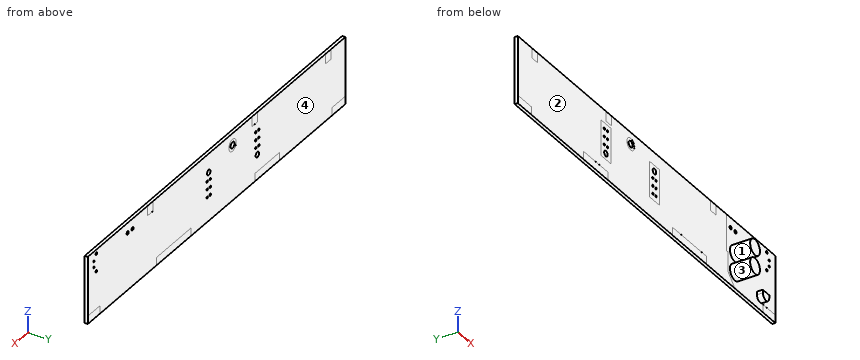
from build123d import *

# Parameters (mm, degrees)
ESQUISSE1_W                     = 210
ESQUISSE1_H                     = 1.6
BOARD_DEPTH                     = 34
SKETCH1_R                       = 0.55
SKETCH1_R_2                     = 1.4
REMOVEABLE_BATT_CON_HOLES_DEPTH = 118.625713289
SKETCH2_R                       = 0.51
SKETCH2_R_2                     = 0.635
DC_OUT_CONN_HOLES_DEPTH         = 118.625713289
SKETCH3_R                       = 0.85
CHARGER_CONN_HOLES_DEPTH        = 118.625713289
SKETCH4_R                       = 1.59
CUT_EXTRUDE1_DEPTH              = 118.625713289
SKETCH5_R                       = 3
SKETCH5_W                       = 10
SKETCH5_H                       = 4
SKETCH5_W_2                     = 28
SKETCH5_W_3                     = 20
SKETCH5_W_4                     = 11
SKETCH5_W_5                     = 4.5
SKETCH5_H_2                     = 5
CUT_EXTRUDE2_DEPTH              = 0.01
CUT_EXTRUDE3_START              = -1.59
SKETCH5_2_R                     = 3
SKETCH5_2_W                     = 10
SKETCH5_2_H                     = 4
SKETCH5_2_W_2                   = 28
SKETCH5_2_W_3                   = 20
SKETCH5_2_W_4                   = 11
SKETCH5_2_W_5                   = 4.5
SKETCH5_2_H_2                   = 5
CUT_EXTRUDE3_DEPTH              = 0.01
SKETCH6_W                       = 8
SKETCH6_H                       = 18
CUT_EXTRUDE4_DEPTH              = 0.001
SKETCH7_R                       = 4
BOSS_EXTRUDE1_DEPTH             = 10.2
BOSS_EXTRUDE2_DEPTH             = 3


with BuildPart() as part:
    # Esquisse1 → Board (new body)
    with BuildSketch(Plane.XY):
        with Locations((-7.593287663, -121.91)):
            Rectangle(ESQUISSE1_W, ESQUISSE1_H)
    extrude(amount=BOARD_DEPTH)

    # Sketch1 → Removeable Batt Con Holes (cut, through all)
    with BuildSketch(Plane(origin=(0, -122.71, 0), x_dir=(1, 0, 0), z_dir=(0, 1, 0))):
        with Locations(Location((-39.523287663, -16.5, 0), (0, 0, 180))):
            Circle(SKETCH1_R)
        with Locations(Location((-42.063287663, -16.5, 0), (0, 0, 180))):
            Circle(SKETCH1_R)
        with Locations(Location((-42.063287663, -20.5, 0), (0, 0, 180))):
            Circle(SKETCH1_R)
        with Locations(Location((-42.063287663, -24.5, 0), (0, 0, 180))):
            Circle(SKETCH1_R)
        with Locations((-40.793287663, -12.5)):
            Circle(SKETCH1_R_2)
        with Locations(Location((-39.523287663, -20.5, 0), (0, 0, 180))):
            Circle(SKETCH1_R)
        with Locations(Location((-39.523287663, -24.5, 0), (0, 0, 180))):
            Circle(SKETCH1_R)
        with Locations(Location((-2.463287663, -20.5, 0), (0, 0, 180))):
            Circle(SKETCH1_R)
        with Locations(Location((0.076712337, -20.5, 0), (0, 0, 180))):
            Circle(SKETCH1_R)
        with Locations(Location((-2.463287663, -16.5, 0), (0, 0, 180))):
            Circle(SKETCH1_R)
        with Locations(Location((0.076712337, -16.5, 0), (0, 0, 180))):
            Circle(SKETCH1_R)
        with Locations(Location((-2.463287663, -12.5, 0), (0, 0, 180))):
            Circle(SKETCH1_R)
        with Locations(Location((0.076712337, -12.5, 0), (0, 0, 180))):
            Circle(SKETCH1_R)
        with Locations((-1.193287663, -24.5)):
            Circle(SKETCH1_R_2)
    extrude(amount=REMOVEABLE_BATT_CON_HOLES_DEPTH, mode=Mode.SUBTRACT)

    # Sketch2 → DC Out Conn holes (cut, through all)
    with BuildSketch(Plane.XZ.offset(122.71)):
        with Locations((92.406712337, 29)):
            Circle(SKETCH2_R)
        with Locations((92.406712337, 26)):
            Circle(SKETCH2_R)
        with Locations((90.446712337, 32)):
            Circle(SKETCH2_R_2)
        with Locations((90.446712337, 23)):
            Circle(SKETCH2_R_2)
    extrude(amount=-DC_OUT_CONN_HOLES_DEPTH, mode=Mode.SUBTRACT)

    # Sketch3 → Charger conn holes (cut, through all)
    with BuildSketch(Plane.XZ.offset(122.71)):
        with Locations((64.906712337, 28.92)):
            Circle(SKETCH3_R)
        with Locations((60.946712337, 28.92)):
            Circle(SKETCH3_R)
    extrude(amount=-CHARGER_CONN_HOLES_DEPTH, mode=Mode.SUBTRACT)

    # Sketch4 → Cut-Extrude1 (cut, through all)
    with BuildSketch(Plane(origin=(0, -121.11, 0), x_dir=(1, 0, 0), z_dir=(0, 1, 0))):
        with Locations(Location((-20.593287663, -28, 0), (0, 0, 180))):
            Circle(SKETCH4_R)
    extrude(amount=-CUT_EXTRUDE1_DEPTH, mode=Mode.SUBTRACT)

    # Sketch5 → Cut-Extrude2 (cut)
    with BuildSketch(Plane(origin=(0, -121.11, 0), x_dir=(1, 0, 0), z_dir=(0, 1, 0))):
        with Locations(Location((-20.593287663, -28, 0), (0, 0, 180))):
            Circle(SKETCH5_R)
        with Locations((92.406712337, -2)):
            Rectangle(SKETCH5_W, SKETCH5_H)
        with Locations((27.406712337, -2)):
            Rectangle(SKETCH5_W_2, SKETCH5_H)
        with Locations((-49.093287663, -2)):
            Rectangle(SKETCH5_W_3, SKETCH5_H)
        with Locations((-107.093287663, -2)):
            Rectangle(SKETCH5_W_4, SKETCH5_H)
        with Locations((-98.743287663, -31.5)):
            Rectangle(SKETCH5_W_5, SKETCH5_H_2)
        with Locations((-38.543287663, -31.5)):
            Rectangle(SKETCH5_W_5, SKETCH5_H_2)
        with Locations((46.656712337, -31.5)):
            Rectangle(SKETCH5_W_5, SKETCH5_H_2)
    extrude(amount=-CUT_EXTRUDE2_DEPTH, mode=Mode.SUBTRACT)

    # Sketch5<2> → Cut-Extrude3 (cut)
    with BuildSketch(Plane(origin=(0, -121.11, 0), x_dir=(1, 0, 0), z_dir=(0, 1, 0)).offset(CUT_EXTRUDE3_START)):
        with Locations(Location((-20.593287663, -28, 0), (0, 0, 180))):
            Circle(SKETCH5_2_R)
        with Locations((92.406712337, -2)):
            Rectangle(SKETCH5_2_W, SKETCH5_2_H)
        with Locations((27.406712337, -2)):
            Rectangle(SKETCH5_2_W_2, SKETCH5_2_H)
        with Locations((-49.093287663, -2)):
            Rectangle(SKETCH5_2_W_3, SKETCH5_2_H)
        with Locations((-107.093287663, -2)):
            Rectangle(SKETCH5_2_W_4, SKETCH5_2_H)
        with Locations((-98.743287663, -31.5)):
            Rectangle(SKETCH5_2_W_5, SKETCH5_2_H_2)
        with Locations((-38.543287663, -31.5)):
            Rectangle(SKETCH5_2_W_5, SKETCH5_2_H_2)
        with Locations((46.656712337, -31.5)):
            Rectangle(SKETCH5_2_W_5, SKETCH5_2_H_2)
    extrude(amount=-CUT_EXTRUDE3_DEPTH, mode=Mode.SUBTRACT)

    # Sketch6 → Cut-Extrude4 (cut)
    with BuildSketch(Plane.XZ.offset(122.71)):
        Polygon((57.406712337, 34), (57.406712337, 15.5), (58.906712337, 15.5), (58.906712337, 5.5), (64.406712337, 0), (41.406712337, 0), (41.406712337, 4), (13.406712337, 4), (13.406712337, 0), (-39.093287663, 0), (-39.093287663, 4), (-59.093287663, 4), (-59.093287663, 0), (-101.593287663, 0), (-101.593287663, 4), (-112.593287663, 4), (-112.593287663, 34), (-100.993287663, 34), (-100.993287663, 29), (-96.493287663, 29), (-96.493287663, 34), (-40.793287663, 34), (-40.793287663, 29), (-36.293287663, 29), (-36.293287663, 34), (44.406712337, 34), (44.406712337, 29), (48.906712337, 29), (48.906712337, 34), align=None)
        with Locations((-40.793287663, 18.5)):
            Rectangle(SKETCH6_W, SKETCH6_H, mode=Mode.SUBTRACT)
        with Locations((-1.193287663, 18.5)):
            Rectangle(SKETCH6_W, SKETCH6_H, mode=Mode.SUBTRACT)
    extrude(amount=-CUT_EXTRUDE4_DEPTH, mode=Mode.SUBTRACT)

    # Sketch7 → Boss-Extrude1 (add)
    with BuildSketch(Plane.XZ.offset(122.71)):
        with Locations(Location((64.406712337, 17.5, 0), (0, 0, 180))):
            Circle(SKETCH7_R)
        with Locations(Location((64.406712337, 8, 0), (0, 0, 180))):
            Circle(SKETCH7_R)
    extrude(amount=BOSS_EXTRUDE1_DEPTH)

    # Sketch8 → Boss-Extrude2 (add)
    with BuildSketch(Plane.XZ.offset(122.71)):
        with BuildLine():
            Line((82.374312337, 7.884), (87.606712337, 7.884))
            Line((87.606712337, 7.884), (87.606712337, 6.354))
            ThreePointArc((87.606712337, 6.354), (84.990512337, 3.7378), (82.374312337, 6.354))
            Line((82.374312337, 6.354), (82.374312337, 7.884))
        make_face()
    extrude(amount=BOSS_EXTRUDE2_DEPTH)


solid = part.part
Build history of the part. All positions in model axes, mm. Face numbers are marked on the shaded views. A direction names the side the tool comes from. Coordinates: 2 decimals unless noted, no trailing zeros. Write each loop counter-clockwise with the first axis right and the second up, starting at its lowest first coordinate (ties: lowest second). Pieces come first, ordered by that corner, then holes.
(1) Mould opens along Z. For the marked faces 1 and 2 say: pulls with the +Z half, pulls with the -Z half, needs draft (parallel to the pull), parting line crosses it, or undercut.
(2) 3-axis set-ups, long thin cutter, end or side, ignore diameter. For the marked faces 3 and 4: which of +Z, -Z, +X, -X, +Y, -Y reach the whole face in a straight line?
(3) Cut at A-A on y = -128.5. List the corners of the cut face in (x, z), and give its area (3 significant figures).
(4) Drill centre lines: line 1 (X direction, y = -122.15, z = 12.5); line 2 (X direction, y = -121.8, z = 24.5); line 3 (X direction, y = -121.7, z = 20.5). Where is each one in solid material? Low to high.
(5) Cut at B-B on x = -79. List the corners of the cut face in (y, z).
(6) Pin check, flat tips, straight feed: pin 1 Ø9.5 at (x, z) = (-20.59, 28) entering from -Y; pin 2 Ø1 at (x, z) = (0.08, 12.5) entering from -Y; pin 3 Ø1.2 at (x, z) = (-105, 2.5) entering from +Y. Stop position of each tip, or through.
Working result:
1. face 1: undercut
1. face 2: needs draft
2. face 3: -Y
2. face 4: +Z, -Z, +X, -X, +Y
3. outline: circle Ø8 at (64.41, 8); circle Ø8 at (64.41, 17.5)
3. area: 101 mm2
4. line 1: x = -112.59 to -42.19, -39.39 to -3.01, -1.91 to -0.47, 0.63 to 97.41
4. line 2: x = -112.59 to -42.61, -41.51 to -40.07, -38.97 to -2.59, 0.21 to 97.41
4. line 3: x = -112.59 to -42.61, -41.51 to -40.07, -38.97 to -3.01, -1.91 to -0.47, 0.63 to 97.41
5. outline: (-122.71, 0) - (-121.11, 0) - (-121.11, 34) - (-122.71, 34) - close
6. pin 1: stops at y = -122.71
6. pin 2: passes through
6. pin 3: stops at y = -121.12
